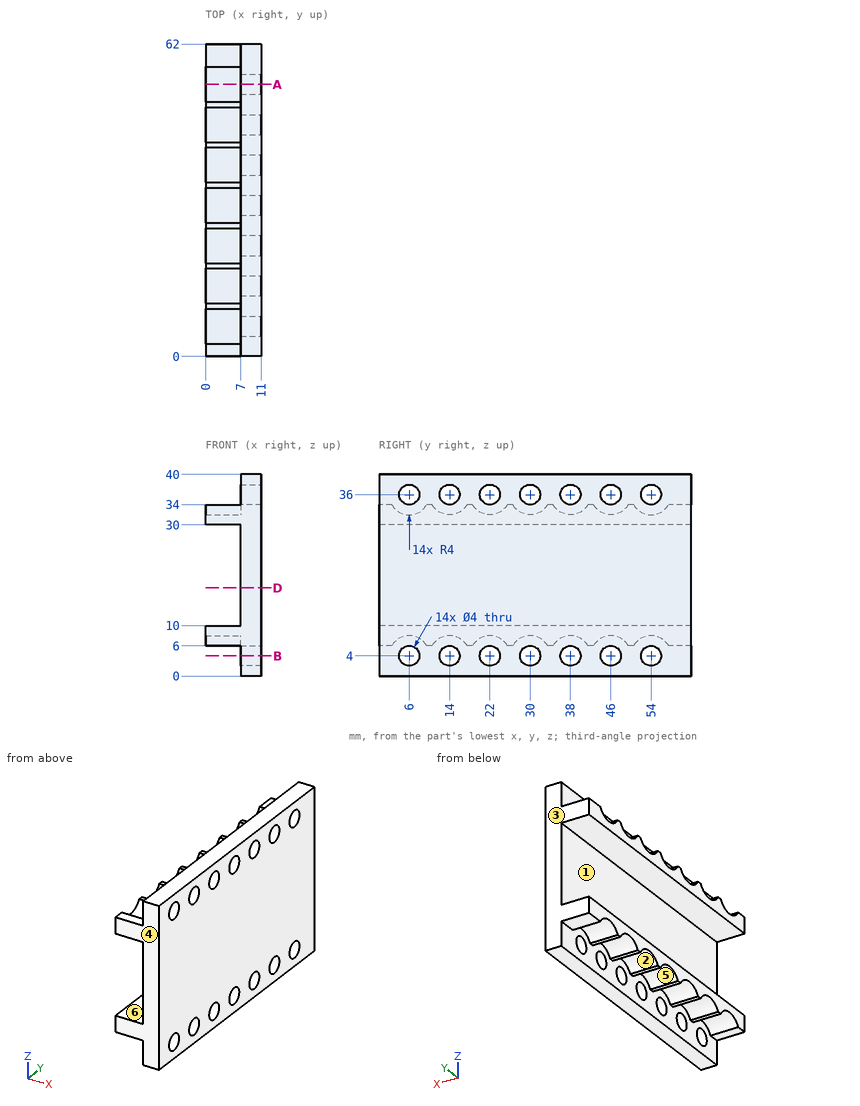
Geometry: see drawing. Coordinates: mm, zero at the bounding-box minimum. A direction names the side the tool comes from. Give positions to 0.01 mm unless a question says otherwise; leave off trailing zeros. Loops run counter-clockwise (first coordinate to the right, second up) from the corner with the lowest first, then second, coordinate; pieces in that order, holes last. Notation, with made-up numbers: (-15.75, 81) - (22.25, 81) arc R19 ccw to (22.25, 111) - close; hole circle Ø7 at (38.5, 33). An arc over 180 degrees is marked (long way). One line per question, with ' | ' between items. Start each with the question number.
(1) Pull-direction query (Z, two-part tool) for the marked faces 1, 2 and 3; classes: released by +Z, released by -Z, zero draft, split by the parting line, or undercut.
(2) Ray query, line 1 (Z direction, x = 8.4, y = 6); line 2 (Z direction, x = 7.5, y = 47); line 3 (X direction, y = 48.5, z = 7). Return the intervals inside material, ascending. Write a range as from..to.
(3) Section query B-B on z = 4. Count the separate pieces of the cut face and the enclosed holes in it, then the cut area to 3 significant figures.
(4) Contact query for flat-ended pins moving along their axis: pin 1 (0.9 mm diameter, centred on x = 3.5, y = 34, fed in from +Z); pin 2 (4 mm diameter, centred on y = 27.5, z = 4, fed in from -X). Output: stop coordinate, or through.
(5) Reachability of the marked faces 4, 5 and 6 from +Z, -Z, +X, -X, +Y, -Y: full face, straight path, thin tool, end or side. Return the list, or none.
(6) Section query A-A on y = 54. Return loops of the section in (x, z), then the cut area to 3 significant figures.
(7) Section query D-D on z = 17.5. Return loops of the section in (x, y).
The answers:
1) face 1: undercut | face 2: released by -Z | face 3: zero draft
2) line 1: 0..2, 6..34, 38..40 | line 2: 0..2.27, 5.73..34.27, 37.73..40 | line 3: 7..11
3) separate pieces: 8 | enclosed holes: 0 | area: 136 mm2
4) pin 1: z = 34 | pin 2: x = 7
5) face 4: +Z, -Z, +X, -X, -Y | face 5: -Z, -X | face 6: -X, +Y, -Y
6) outline: (0, 8) - (7, 8) - (7, 6) - (11, 6) - (11, 34) - (7, 34) - (7, 32) - (0, 32) - (0, 30) - (7, 30) - (7, 10) - (0, 10) - close; (7, 0) - (11, 0) - (11, 2) - (7, 2) - close; (7, 38) - (11, 38) - (11, 40) - (7, 40) - close | area: 156 mm2
7) outline: (7, 0) - (11, 0) - (11, 62) - (7, 62) - close
